from build123d import *

# Parameters (mm, degrees)
BOSS_SWITCH_BODY_DEPTH                    = 3
SKETCH1_W                                 = 4
SKETCH1_H                                 = 3.5
BOSS_FLANGE_WIDTH_DEPTH                   = 5
BOSS_FLANGE_HEIGHT_REACH                  = 35.863
SKETCH2_W                                 = 4
SKETCH2_H                                 = 2
SKETCH2_W_2                               = 8
CUT_UP_TO_DOWN_DERAILLEUR_CLEARANCE_REACH = 21.462
SKETCH10_W                                = 2.453096586
SKETCH10_H                                = 3
SKETCH17_W                                = 12.1675
SKETCH17_H                                = 4
BOSS_FLANGE_SUPPORT_DEPTH                 = 14.5
TAP_DRILL_FOR_M2X0_4_TAP1_D               = 1.6
M2_CLEARANCE_HOLE2_D                      = 2.4
M2_CLEARANCE_HOLE2_DEPTH                  = 15
M2_CLEARANCE_HOLE2_TIP                    = 0.721032743
CHAMFER_FLANGE_SUPPORT_SIZE               = 1.5
CHAMFER_FLANGE_SUPPORT_2_SIZE             = 1.5
CHAMFER_FLANGE_SUPPORT_3_SIZE             = 1
SKETCH23_W                                = 3.9675
SKETCH23_H                                = 12
CUT_GAP_FOR_PRINTING_DEPTH                = 32.000499688
SKETCH25_W                                = 0.953096586
SKETCH25_H                                = 3.5
CUT_DERAILLEUR_CLEARANCE_DEPTH            = 32.145320369
CHAMFER8_SIZE                             = 1
CUT_EXTRUDE1_REACH                        = 30.441
SKETCH26_W                                = 7.075346244
SKETCH26_H                                = 3.905124838
CUT_WIDE_DERAILLEUR_CLEARANCE_DEPTH       = 33.195879702
CUT_WIDE_DERAILLEUR_CLEARANCE_DEPTH_BACK  = 4
SKETCH27_W                                = 2
SKETCH27_H                                = 5
CHAMFER9_SIZE                             = 1


# Some blends are built 0.0001 mm under size
with BuildPart() as part:
    # Sketch-SwitchBossUp → Boss-Switch Body (new body)
    with BuildSketch(Plane.XY):
        with BuildLine():
            Line((5.581091201, 12.555245643), (5.581100766, 11.263016279))
            Line((5.581100766, 11.263016279), (3.971265023, 11.263016279))
            Line((3.971265023, 11.263016279), (3.971265023, 11.909403061))
            Line((3.971265023, 11.909403061), (3.296271341, 11.909403061))
            Line((3.296271341, 11.909403061), (3.296271341, 11.409403061))
            Line((3.296271341, 11.409403061), (3.296271341, 9.409403061))
            Line((3.296271341, 9.409403061), (3.296271341, 8.909403061))
            Line((3.296271341, 8.909403061), (3.971278743, 8.519687356))
            Line((3.971278743, 8.519687356), (3.971278743, 9.409408058))
            Line((3.971278743, 9.409408058), (5.815189336, 10.763016279))
            Line((5.815189336, 10.763016279), (6.627976927, 9.860324207))
            Line((6.627976927, 9.860324207), (6.627976927, 8.210536506))
            Line((6.627976927, 8.210536506), (5.581127833, 7.606137899))
            Line((5.581127833, 7.606137899), (4.906138119, 7.216432406))
            Line((4.906138119, 7.216432406), (4.906138119, 5.216432406))
            Line((4.906138119, 5.216432406), (5.58114552, 4.826716701))
            Line((5.58114552, 4.826716701), (6.342350466, 4.826716701))
            Line((6.342350466, 4.826716701), (6.342350466, 4.326716701))
            Line((6.342350466, 4.326716701), (5.374946804, 3.937018274))
            Line((5.374946804, 3.937018274), (4.374946804, 3.937018274))
            Line((4.374946804, 3.937018274), (5.038286759, 1.461399857))
            Line((5.038286759, 1.461399857), (6.03883266, 0.837018274))
            Line((6.03883266, 0.837018274), (6.627976927, 0.837018274))
            Line((6.627976927, 0.837018274), (6.627976927, -1.165310653))
            Line((6.627976927, -1.165310653), (5.038286759, -1.165310653))
            Line((5.038286759, -1.165310653), (3.03883266, -1.165310653))
            Line((3.03883266, -1.165310653), (3.03883266, 0.834689347))
            Line((3.03883266, 0.834689347), (4.03855971, 1.460381193))
            Line((4.03855971, 1.460381193), (3.374946804, 3.937018274))
            Line((3.374946804, 3.937018274), (2.842350466, 4.326720436))
            Line((2.842350466, 4.326720436), (2.842350466, 4.826720436))
            Line((2.842350466, 4.826720436), (3.58114552, 4.826720436))
            Line((3.58114552, 4.826720436), (4.256138119, 5.216427595))
            Line((4.256138119, 5.216427595), (4.256138119, 7.216427595))
            Line((4.256138119, 7.216427595), (3.581130717, 7.6061433))
            Line((3.581130717, 7.6061433), (2.9061262, 7.216422599))
            Line((2.9061262, 7.216422599), (0.971281627, 7.216422599))
            Line((0.971281627, 7.216422599), (0.971281627, 9.019692757))
            Line((0.971281627, 9.019692757), (1.971281627, 9.019692757))
            Line((1.971281627, 9.019692757), (2.646271341, 9.40939825))
            Line((2.646271341, 9.40939825), (2.646271341, 11.40939825))
            Line((2.646271341, 11.40939825), (0.897326855, 12.41915182))
            Line((0.897326855, 12.41915182), (0.545466745, 12.771663724))
            Line((0.545466745, 12.771663724), (-0.372784255, 18.226393961))
            ThreePointArc((-0.372784255, 18.226393961), (-0.209313172, 18.996084896), (0.435897335, 19.446473985))
            Line((0.435897335, 19.446473985), (-0.46073685, 24.772792819))
            ThreePointArc((-0.46073685, 24.772792819), (-2.630501593, 26.270619745), (-2.852546321, 28.897797067))
            ThreePointArc((-2.852546321, 28.897797067), (-1.887813913, 29.338582026), (-1.447028953, 28.373849618))
            ThreePointArc((-1.447028953, 28.373849618), (-0.703448682, 26.416936722), (1.333779254, 26.898727173))
            ThreePointArc((1.333779254, 26.898727173), (2.379722745, 27.074801628), (2.555797201, 26.028858137))
            ThreePointArc((2.555797201, 26.028858137), (2.086504637, 25.507104397), (1.511513111, 25.104801997))
            Line((1.511513111, 25.104801997), (1.553598189, 24.854801997))
            Line((1.553598189, 24.854801997), (9.027976927, 24.854801997))
            Line((9.027976927, 24.854801997), (9.027976927, 22.354801997))
            Line((9.027976927, 22.354801997), (1.974448974, 22.354801997))
            Line((1.974448974, 22.354801997), (3.516958068, 13.191761617))
            Line((3.516958068, 13.191761617), (3.808459197, 12.945132837))
            Line((3.808459197, 12.945132837), (4.256080915, 12.944958203))
            Line((4.256080915, 12.944958203), (4.791964496, 14.944962169))
            Line((4.791964496, 14.944962169), (4.116925685, 15.334689347))
            Line((4.116925685, 15.334689347), (3.581073513, 15.334689347))
            Line((3.581073513, 15.334689347), (3.581073513, 18.834689347))
            Line((3.581073513, 18.834689347), (5.725580434, 18.834689347))
            Line((5.725580434, 18.834689347), (6.627976927, 18.834689347))
            Line((6.627976927, 18.834689347), (6.627976927, 15.334689347))
            Line((6.627976927, 15.334689347), (6.116971898, 15.334689347))
            Line((6.116971898, 15.334689347), (5.441964496, 14.94496698))
            Line((5.441964496, 14.94496698), (4.906080915, 12.944963014))
            Line((4.906080915, 12.944963014), (5.581091201, 12.555245643))
        make_face()
    extrude(amount=BOSS_SWITCH_BODY_DEPTH)

    # Sketch1 → Boss-Flange Width (add)
    with BuildSketch(Plane(origin=(0, 0, 0), x_dir=(-1, 0, 0), z_dir=(0, 0, -1))):
        Polygon((-7.581073513, -1.165310653), (0.412170615, -1.165310653), (0.412170615, 0.834689347), (-3.03883266, 0.834689347), (-4.03855971, 1.460381193), (-5.03855971, 1.460381193), (-6.03883266, 0.837018274), (-7.581073513, 0.837018274), align=None)
        with Locations((-5.581073513, 17.084689347)):
            Rectangle(SKETCH1_W, SKETCH1_H)
    extrude(amount=BOSS_FLANGE_WIDTH_DEPTH)

    # Sketch2 → Boss-Flange Height (add, up to next)
    with BuildSketch(Plane(origin=(-7.039523073, 0, 0), x_dir=(0, 0, -1), z_dir=(1, 0, 0)), mode=Mode.PRIVATE) as boss_flange_height_sk1:
        with Locations((3, 16.334689347)):
            Rectangle(SKETCH2_W, SKETCH2_H)
    boss_flange_height_tool1 = extrude(boss_flange_height_sk1.sketch, amount=BOSS_FLANGE_HEIGHT_REACH, mode=Mode.PRIVATE) - part.part
    # Sketch2 → Boss-Flange Height (add, up to next)
    with BuildSketch(Plane(origin=(-7.039523073, 0, 0), x_dir=(0, 0, -1), z_dir=(1, 0, 0)), mode=Mode.PRIVATE) as boss_flange_height_sk2:
        with Locations((1, -0.165310653)):
            Rectangle(SKETCH2_W_2, SKETCH2_H)
    boss_flange_height_tool2 = extrude(boss_flange_height_sk2.sketch, amount=BOSS_FLANGE_HEIGHT_REACH, mode=Mode.PRIVATE) - part.part
    add(boss_flange_height_tool1.solids().sort_by_distance((-7.039523, 16.334689, -3))[0])
    add(boss_flange_height_tool2.solids().sort_by_distance((-7.039523, -0.165311, -1))[0])

    # Sketch10 → Cut-Up-To-Down Derailleur Clearance (cut, up to next)
    with BuildSketch(Plane(origin=(0, 15.334689347, 0), x_dir=(1, 0, 0), z_dir=(0, 1, 0)), mode=Mode.PRIVATE) as cut_up_to_down_derailleur_clearance_sk1:
        with Locations((6.35452522, 3.5)):
            Rectangle(SKETCH10_W, SKETCH10_H)
    cut_up_to_down_derailleur_clearance_tool1 = extrude(cut_up_to_down_derailleur_clearance_sk1.sketch, amount=CUT_UP_TO_DOWN_DERAILLEUR_CLEARANCE_REACH, mode=Mode.PRIVATE) & part.part
    add(cut_up_to_down_derailleur_clearance_tool1.solids().sort_by_distance((6.354525, 15.334689, -3.5))[0], mode=Mode.SUBTRACT)

    # Sketch17 → Boss-Flange Support (add)
    with BuildSketch(Plane.XZ.offset(-15.334689347)):
        with Locations((-0.955773073, -3)):
            Rectangle(SKETCH17_W, SKETCH17_H)
    extrude(amount=BOSS_FLANGE_SUPPORT_DEPTH)

    # Tap Drill for M2x0.4 Tap1 (through all)
    with Locations(Plane(origin=(0, -1.165310653, 0), x_dir=(-1, 0, 0), z_dir=(0, -1, 0))):
        with Locations((5.039523073, 3), (0.539523073, 3)):
            Hole(TAP_DRILL_FOR_M2X0_4_TAP1_D / 2)

    # M2 Clearance Hole2
    with Locations(Plane.XZ.offset(1.165310653)):
        with Locations((-5.039523073, -3), (-0.539523073, -3)):
            Hole(M2_CLEARANCE_HOLE2_D / 2, depth=M2_CLEARANCE_HOLE2_DEPTH)
            with Locations((0, 0, -(M2_CLEARANCE_HOLE2_DEPTH + M2_CLEARANCE_HOLE2_TIP / 2))):  # 118° drill point
                Cone(0, M2_CLEARANCE_HOLE2_D / 2, M2_CLEARANCE_HOLE2_TIP, mode=Mode.SUBTRACT)

    # Chamfer-Flange Support
    chamfer_flange_support_edges = [part.edges().sort_by_distance(p)[0] for p in [
        (3.581073513, 17.334689347, -3),
    ]]
    chamfer(chamfer_flange_support_edges, length=CHAMFER_FLANGE_SUPPORT_SIZE - 0.0001)  # a hair under: the kernel refuses the full size

    # Chamfer-Flange Support 2
    chamfer_flange_support_2_edges = [part.edges().sort_by_distance(p)[0] for p in [
        (5.127976927, 17.084689347, -2),
        (5.127976927, 15.334689347, -1.5),
    ]]
    chamfer(chamfer_flange_support_2_edges, length=CHAMFER_FLANGE_SUPPORT_2_SIZE)

    # Chamfer-Flange Support 3
    chamfer_flange_support_3_edges = [part.edges().sort_by_distance(p)[0] for p in [
        (-2.000345206, 0.834689347, -1),
    ]]
    chamfer(chamfer_flange_support_3_edges, length=CHAMFER_FLANGE_SUPPORT_3_SIZE)

    # Sketch23 → Cut-Gap for Printing (cut, through all)
    with BuildSketch(Plane.XY.offset(-1)):
        with Locations((3.144226927, 7.834689347)):
            Rectangle(SKETCH23_W, SKETCH23_H)
    extrude(amount=-CUT_GAP_FOR_PRINTING_DEPTH, mode=Mode.SUBTRACT)

    # Sketch25 → Cut-Derailleur Clearance (cut, through all)
    with BuildSketch(Plane.XY):
        with Locations((7.10452522, 17.084689347)):
            Rectangle(SKETCH25_W, SKETCH25_H)
    extrude(amount=-CUT_DERAILLEUR_CLEARANCE_DEPTH, mode=Mode.SUBTRACT)

    # Chamfer8
    # the kernel refuses this chamfer: 1 mm, written as the material it adds along each edge
    with BuildSketch(Plane(origin=(6.627976927, 0.837018274, 0), x_dir=(-0.027495876610586494, 0, 0.9996219169112968), z_dir=(0, -1, 0))) as chamfer8_piece_1_section:
        Polygon((CHAMFER8_SIZE * 0.999621916911, -CHAMFER8_SIZE * 0.0274958766106), (-CHAMFER8_SIZE * 0.0274958766106, -CHAMFER8_SIZE * 0.999621916911), (0, 0), align=None)
    chamfer8_piece_1 = extrude(amount=2.002328927, mode=Mode.PRIVATE)
    chamfer8_piece_1 = split(chamfer8_piece_1, bisect_by=Plane(origin=(7.581073513, -0.16414619, 0.332375145), z_dir=(-1, 0, 0)), keep=Keep.TOP, mode=Mode.PRIVATE)
    add(chamfer8_piece_1)

    # Sketch26 → Cut-Extrude1 (cut, up to next)
    with BuildSketch(Plane(origin=(-5.954769273, 8.400426305, 7.000355254), x_dir=(-0.8782236755158304, -0.3674019179359696, -0.30616826494664123), z_dir=(0.47825011841448156, -0.6746701157774819, -0.5622250964812346)), mode=Mode.PRIVATE) as cut_extrude1_sk1:
        with Locations((-16.492565132, 13.959094076)):
            Rectangle(SKETCH26_W, SKETCH26_H)
    cut_extrude1_tool1 = extrude(cut_extrude1_sk1.sketch, amount=CUT_EXTRUDE1_REACH, mode=Mode.PRIVATE) & part.part
    add(cut_extrude1_tool1.solids().sort_by_distance((8.529392, 23.396221, 1.326182))[0], mode=Mode.SUBTRACT)

    # Sketch27 → Cut-Wide Derailleur Clearance (cut, two sides: drawn at the far end of the back side and taken through both)
    with BuildSketch(Plane(origin=(5.127976927, 0, 0), x_dir=(0, 0, -1), z_dir=(1, 0, 0)).offset(-CUT_WIDE_DERAILLEUR_CLEARANCE_DEPTH_BACK)):
        with Locations((4, 16.334689347)):
            Rectangle(SKETCH27_W, SKETCH27_H)
    extrude(amount=CUT_WIDE_DERAILLEUR_CLEARANCE_DEPTH + CUT_WIDE_DERAILLEUR_CLEARANCE_DEPTH_BACK, mode=Mode.SUBTRACT)

    # Chamfer9
    chamfer9_edges = [part.edges().sort_by_distance(p)[0] for p in [
        (4.60452522, 18.834689347, -3),
    ]]
    chamfer(chamfer9_edges, length=CHAMFER9_SIZE)


solid = part.part
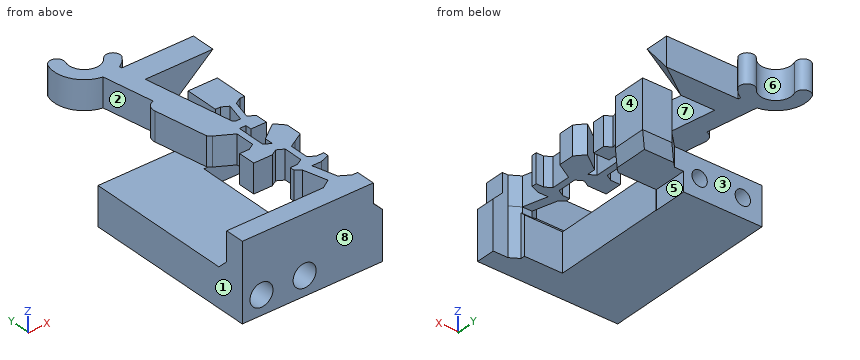
Could you check a few things on this model? Use its own coordinates, in mm. Face numbers are marked on the shaded views. A direction names the side the tool comes from. Coordinates: 2 decimals unless noted, no trailing zeros. Order: outer loops, then holes, each group sorted by start corner. A loop starts at its lowest first (then second) coordinate and runs counter-clockwise, first axis right, second up. Notation, with made-up numbers: (-26.5, 76) -> (26.5, 76) arc R27 cw to (26.5, 114) -> close; hole circle Ø6 at (-37.5, 73). An arc over 180 degrees is marked (long way). One line per item, written item: value. Start each with the question number.
1) Which directions (+Z, -Z, +X, -X, +Y, -Y) give clear straight access to the entire face, cutting with the end or side of a thin tool? Please do the marked faces 1, 2, 3 and 4.
2) If I drill on L1, parallel to X at y = 9.75, z = -3; L2, parallel to X at y = 8.5, z = -2.25; L3, parallel to Y at x = 0, z = -1.25, over which ranges is the centre line in solid material (lowest first)? Write a range as [from, to].
3) Imagine slicing it at B-B on y = 23.5. List the corners of the cut face in (x, z) for me, plus the area to 3 significant figures.
4) I'm going to push flat-ended pins straight in: pin 1 (1.6 mm diameter, centred on y = 10, z = 2, fed in from -X); pin 2 (0.6 mm diameter, centred on y = -0.5, z = -2.5, fed in from +X); pin 3 (1.8 mm diameter, centred on y = 17.5, z = 1.5, fed in from -X); pin 4 (6 mm diameter, centred on x = 1, y = 19.5, fed in from -Z). Where does each tip first touch, or does it pass through?
5) We'd pull the mould along X, two halves only. Please class the marked faces 5, 6, 7 and 8: +X half, -X half, draft (parallel to the pull), parting line (faces both ways), or undercut.
6) Imagine slicing it at C-C on y = 20. List the corners of the cut face in (x, z) for me.
7) Imagine slicing it at A-A on z = -2.5. Count the separate pieces of the cut face and the enclosed holes in it, plus the area to 3 significant figures.
Answer list:
1. face 1: +Z, -Z, -X, +Y, -Y
1. face 2: +Z, -Z, -X
1. face 3: -Z, -X, +Y
1. face 4: +Z, -Z, +X
2. L1: x = [-7.04, -6.24], [-3.84, -1.74], [0.66, 1.16]
2. L2: x = [-7.04, -5.98], [-4.1, -1.48], [0.4, 1.16]
2. L3: y = [-1.17, 17.33]
3. outline: (-0.25, 0) -> (7.12, 0) -> (9.03, 1.63) -> (9.03, 3) -> (-0.25, 3) -> close
3. area: 26.3 mm2
4. pin 1: stops at x = 2.28
4. pin 2: stops at x = 7.58
4. pin 3: stops at x = -0.39
4. pin 4: stops at z = -5
5. face 5: +X half
5. face 6: undercut
5. face 7: undercut
5. face 8: draft
6. outline: (0.34, 0) -> (2.37, 0) -> (2.37, 3) -> (0.34, 3) -> close
7. separate pieces: 3
7. enclosed holes: 0
7. area: 115 mm2
